from build123d import *

# Parameters (mm, degrees)
CROQUIS1_R              = 120
SALIENTE_EXTRUIR1_DEPTH = 6.5
CROQUIS2_R              = 4
CORTAR_EXTRUIR1_DEPTH   = 6.5
CROQUIS3_R              = 3.175
CORTAR_EXTRUIR2_DEPTH   = 6.5
CROQUIS4_R              = 1.5
CORTAR_EXTRUIR3_DEPTH   = 10


with BuildPart() as part:
    # Croquis1 → Saliente-Extruir1 (new body)
    with BuildSketch(Plane(origin=(0, 0, 0), x_dir=(1, 0, 0), z_dir=(0, 1, 0))):
        with Locations(Location((0, 0, 0), (0, 0, 270))):
            Circle(CROQUIS1_R)
    extrude(amount=SALIENTE_EXTRUIR1_DEPTH)

    # Croquis2 → Cortar-Extruir1 (cut)
    with BuildSketch(Plane(origin=(0, 6.5, 0), x_dir=(1, 0, 0), z_dir=(0, 1, 0))):
        with Locations(Location((0, 0, 0), (0, 0, 270))):
            Circle(CROQUIS2_R)
    extrude(amount=-CORTAR_EXTRUIR1_DEPTH, mode=Mode.SUBTRACT)

    # Croquis3 → Cortar-Extruir2 (cut)
    with BuildSketch(Plane(origin=(0, 0, 0), x_dir=(-1, 0, 0), z_dir=(0, -1, 0))):
        with Locations(Location((-28.4, 0, 0), (0, 0, 90))):
            Circle(CROQUIS3_R)
        with Locations(Location((-56.8, 0, 0), (0, 0, 90))):
            Circle(CROQUIS3_R)
        with Locations(Location((-85.2, 0, 0), (0, 0, 90))):
            Circle(CROQUIS3_R)
        with Locations(Location((85.2, 0, 0), (0, 0, 270))):
            Circle(CROQUIS3_R)
        with Locations(Location((56.8, 0, 0), (0, 0, 270))):
            Circle(CROQUIS3_R)
        with Locations(Location((28.4, 0, 0), (0, 0, 270))):
            Circle(CROQUIS3_R)
        with Locations(Location((0, -28.4, 0), (0, 0, 90))):
            Circle(CROQUIS3_R)
        with Locations(Location((0, -56.8, 0), (0, 0, 90))):
            Circle(CROQUIS3_R)
        with Locations(Location((0, -85.2, 0), (0, 0, 90))):
            Circle(CROQUIS3_R)
        with Locations(Location((0, 85.2, 0), (0, 0, 270))):
            Circle(CROQUIS3_R)
        with Locations(Location((0, 56.8, 0), (0, 0, 270))):
            Circle(CROQUIS3_R)
        with Locations(Location((0, 28.4, 0), (0, 0, 270))):
            Circle(CROQUIS3_R)
    extrude(amount=-CORTAR_EXTRUIR2_DEPTH, mode=Mode.SUBTRACT)

    # Croquis4 → Cortar-Extruir3 (cut)
    with BuildSketch(Plane.XZ):
        with Locations(Location((20, -99.505571576, 0), (0, 0, 270))):
            Circle(CROQUIS4_R)
        with Locations(Location((-20, -99.505571576, 0), (0, 0, 90))):
            Circle(CROQUIS4_R)
        with Locations(Location((-96.174352803, 32.432277712, 0), (0, 0, 270))):
            Circle(CROQUIS4_R)
        with Locations(Location((-76.174352803, 67.073293864, 0), (0, 0, 90))):
            Circle(CROQUIS4_R)
        with Locations(Location((76.174352803, 67.073293864, 0), (0, 0, 270))):
            Circle(CROQUIS4_R)
        with Locations(Location((96.174352803, 32.432277712, 0), (0, 0, 90))):
            Circle(CROQUIS4_R)
    extrude(amount=-CORTAR_EXTRUIR3_DEPTH, mode=Mode.SUBTRACT)


solid = part.part
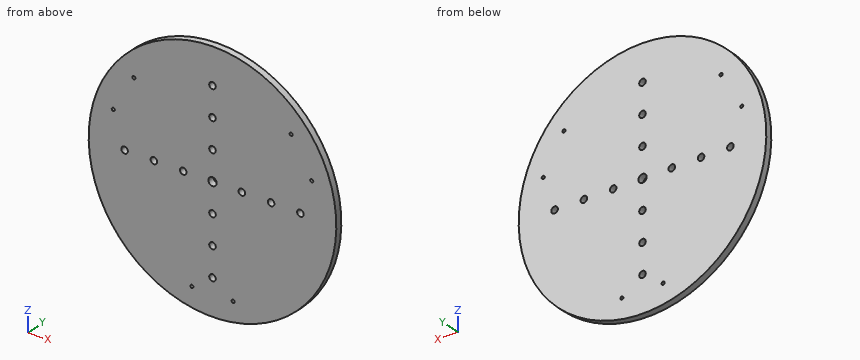
Could you check a few things on this model? Use its own coordinates, in mm. Give positions to 0.01 mm unless a question says otherwise; leave off trailing zeros. Loops run counter-clockwise (first coordinate to the right, second up) from the corner with the lowest first, then second, coordinate; pieces in that order, holes last. Notation, with made-up numbers: M 75.5,77 L 90.5,77 A19 cw 90.5,94 Z; hole C 9,85.25 d6. An arc over 180 degrees is marked long. Answer as a JSON object with one key per item and string values.
Q1. Suppose I cut it at D-D, the plane z = -63.5. List the corners of the cut face in (x, y) for me.
Values found:
{"outline": "M -101.82,0 L 101.82,0 L 101.82,6.5 L -101.82,6.5 Z"}
Q2. If I drill on probe 1 along Z at (x, y) = (-26, 5.5); probe 2 along Z at (x, y) = (18, 1.75); probe 3 along X at (y, z) = (5, -28.4) (3 decimals), over which ranges is the centre line in solid material (lowest first)? Write a range as [from, to].
Values found:
{"probe 1": "z = [-117.15, -2.08], [2.08, 117.15]", "probe 2": "z = [-118.64, 118.64]", "probe 3": "x = [-116.591, -3.175], [3.175, 116.591]"}
Q3. Suppose I cut it at B-B, the plane z = 85.2. List the corners of the cut face in (x, y) for me (3 decimals), plus the area to 3 significant figures.
Values found:
{"outline": "M -84.504,0 L -3.175,0 L -3.175,6.5 L -84.504,6.5 Z; M 3.175,0 L 84.504,0 L 84.504,6.5 L 3.175,6.5 Z", "area": "1,060 mm²"}
Q4. For P1, Ø2.5, axis at x = 76.17, z = 67.07, coming from the -Y side; P2, Ø1.5, axis at x = -74.5, y = 4, coming from the -Z side; P3, Ø1.5, axis at x = 35, y = 5.5, coming from the -Z side, each with a flat end and sliding along its axis, tell me the tip position at first contact or that it passes through.
Values found:
{"P1": "passes through", "P2": "stops at z = -94.66", "P3": "stops at z = -115.01"}
Q5. Suppose I cut it at C-C, the plane y = 2.5. State how many separate pieces and enclosed holes the cut face has, plus the area to 3 significant figures.
Values found:
{"separate pieces": "1", "enclosed holes": "19", "area": "44,800 mm²"}
Q6. Suppose I cut it at A-A, the plane x = -28.4. List the corners of the cut face in (y, z) for me (3 decimals).
Values found:
{"outline": "M 0,-116.591 L 6.5,-116.591 L 6.5,-3.175 L 0,-3.175 Z; M 0,3.175 L 6.5,3.175 L 6.5,116.591 L 0,116.591 Z"}
